Source: CAD feature listing. Evaluate the final solid. Frame: model axes, mm. A direction names the side the tool comes from. Coordinates: 2 decimals unless noted, no trailing zeros. Write each loop counter-clockwise with the first axis right and the second up, starting at its lowest first coordinate (ties: lowest second). Pieces come first, ordered by that corner, then holes. Notation, with made-up numbers: (48.25, 15.25) -> (58.25, 15.25) arc R26 cw to (58.25, 51.25) -> close; hole circle Ø2 at (-30, 77). An arc over 180 degrees is marked (long way). Write item = value, one per line.
from build123d import *

# Parameters (mm, degrees)
SKETCH1_R          = 13.5
EXTRUDE1_DEPTH     = 4
SKETCH3_R          = 10
EXTRUDE3_DEPTH     = 25
SKETCH7_R          = 8.5
CUT_EXTRUDE5_DEPTH = 16
SKETCH4_R          = 7.5
EXTRUDE4_DEPTH     = 14
CHAMFER1_SIZE      = 0.2
CHAMFER3_SIZE      = 0.3
SKETCH5_R          = 12
SKETCH5_R_2        = 10
CUT_EXTRUDE1_DEPTH = 1.5
SKETCH8_R          = 8
CUT_EXTRUDE6_DEPTH = 2
CHAMFER5_SIZE      = 1
SKETCH6_R          = 0.65
CUT_EXTRUDE2_DEPTH = 5
CHAMFER6_SIZE      = 0.2
EXTRUDE5_DEPTH     = 4


with BuildPart() as part:
    # Sketch1 → Extrude1 (new body)
    with BuildSketch(Plane.XY):
        Circle(SKETCH1_R)
    extrude(amount=EXTRUDE1_DEPTH)

    # Sketch3 → Extrude3 (add)
    with BuildSketch(Plane(origin=(0, 0, 0), x_dir=(-1, 0, 0), z_dir=(0, 0, -1))):
        Circle(SKETCH3_R)
    extrude(amount=EXTRUDE3_DEPTH)

    # Sketch7 → Cut-Extrude5 (cut)
    with BuildSketch(Plane.XY.offset(4)):
        Circle(SKETCH7_R)
    extrude(amount=-CUT_EXTRUDE5_DEPTH, mode=Mode.SUBTRACT)

    # Sketch4 → Extrude4 (add)
    with BuildSketch(Plane.XY.offset(-12)):
        Circle(SKETCH4_R)
    extrude(amount=EXTRUDE4_DEPTH)

    # Chamfer1
    chamfer1_edges = [part.edges().sort_by_distance(p)[0] for p in [
        (-7.5, 0, 2),
    ]]
    chamfer(chamfer1_edges, length=CHAMFER1_SIZE)

    # Chamfer3
    chamfer3_edges = [part.edges().sort_by_distance(p)[0] for p in [
        (-8.5, 0, 4),
        (-13.5, 0, 4),
    ]]
    chamfer(chamfer3_edges, length=CHAMFER3_SIZE)

    # Sketch5 → Cut-Extrude1 (cut)
    with BuildSketch(Plane(origin=(0, 0, 0), x_dir=(-1, 0, 0), z_dir=(0, 0, -1))):
        Circle(SKETCH5_R)
        Circle(SKETCH5_R_2, mode=Mode.SUBTRACT)
    extrude(amount=-CUT_EXTRUDE1_DEPTH, mode=Mode.SUBTRACT)

    # Sketch8 → Cut-Extrude6 (cut)
    with BuildSketch(Plane(origin=(0, 0, -25), x_dir=(-1, 0, 0), z_dir=(0, 0, -1))):
        Circle(SKETCH8_R)
    extrude(amount=-CUT_EXTRUDE6_DEPTH, mode=Mode.SUBTRACT)

    # Chamfer5
    chamfer5_edges = [part.edges().sort_by_distance(p)[0] for p in [
        (10, 0, -25),
    ]]
    chamfer(chamfer5_edges, length=CHAMFER5_SIZE)

    # Sketch6 → Cut-Extrude2 (cut)
    with BuildSketch(Plane.XY.offset(2)):
        with Locations((1.500332219, -0.655252352)):
            Circle(SKETCH6_R)
        with Locations((0, 2.126873458)):
            Circle(SKETCH6_R)
        with Locations((0, -4.848601397)):
            Circle(SKETCH6_R)
        with Locations((2.83413915, -3.376897165)):
            Circle(SKETCH6_R)
        with Locations((1.947084544, 4.606594287)):
            Circle(SKETCH6_R)
        with Locations((4.971134337, -0.373007704)):
            Circle(SKETCH6_R)
        with Locations((-4.084079731, 2.409118105)):
            Circle(SKETCH6_R)
        with Locations((-4.971134337, -0.373007704)):
            Circle(SKETCH6_R)
        with Locations((-1.947084544, 4.606594287)):
            Circle(SKETCH6_R)
        with Locations((-2.83413915, -3.376897165)):
            Circle(SKETCH6_R)
        with Locations((-1.500332219, -0.655252352)):
            Circle(SKETCH6_R)
        with Locations((4.084079731, 2.409118105)):
            Circle(SKETCH6_R)
    extrude(amount=-CUT_EXTRUDE2_DEPTH, mode=Mode.SUBTRACT)

    # Chamfer6
    chamfer6_edges = [part.edges().sort_by_distance(p)[0] for p in [
        (0.850332219, -0.655252352, 2),
        (-0.65, 2.126873458, 2),
        (-0.65, -4.848601397, 2),
        (1.297084544, 4.606594287, 2),
        (2.18413915, -3.376897165, 2),
        (4.321134337, -0.373007704, 2),
        (-4.734079731, 2.409118105, 2),
        (-5.621134337, -0.373007704, 2),
        (-2.597084544, 4.606594287, 2),
        (-3.48413915, -3.376897165, 2),
        (-2.150332219, -0.655252352, 2),
        (3.434079731, 2.409118105, 2),
    ]]
    chamfer(chamfer6_edges, length=CHAMFER6_SIZE)

    # Sketch9 → Extrude5 (add)
    with BuildSketch(Plane(origin=(0, 0, -23), x_dir=(-1, 0, 0), z_dir=(0, 0, -1))):
        Polygon((-7.216878365, 12.5), (7.216878365, 12.5), (14.43375673, 0), (7.216878365, -12.5), (-7.216878365, -12.5), (-14.43375673, 0), align=None)
    extrude(amount=-EXTRUDE5_DEPTH)


solid = part.part
1) Pull-direction query (Y, two-part tool) for faces 4 (the flat face through (7.4, -7.3, -23)), 5 (the cylindrical face through (2.17, -9.76, -23.51)), 6 (the flat face through (3, -3, -3)), 7 (the flat face through (10.775, -6.337, -21.028)); classes: +Y half, -Y half, draft (parallel to the pull), parting line (faces both ways), or undercut.
Answer block:
face_4 = draft
face_5 = parting line
face_6 = undercut
face_7 = -Y half
2) Reachability of faces 1 (the cylindrical face through (2.17, -9.76, -8.89)), 2 (the flat face through (-4, 2, -3)), 3 (the flat face through (-10.876, -6.163, -21.028)) from +Z, -Z, +X, -X, +Y, -Y: full face, straight path, thin tool, end or side. Return the list, or none.
Answer block:
face_1 = none
face_2 = +Z
face_3 = -Z, -X, -Y
3) First-contact query: pin 1 Ø12 at (y, z) = (-4.5, -10) entering from -X; pin 2 Ø2 at (x, y) = (-1.95, 4.61) entering from +Z; pin 3 Ø6 at (x, y) = (-11, 6.5) entering from -Z. Flat tips, straight axial feed; report the tip coordinate or a pass-through.
Answer block:
pin_1 = -10
pin_2 = 2
pin_3 = -24.22
4) Cut plane A-A, the plane z = -20.25. Output: boundary loops of the cut face in (x, y), and give its area (3 significant figures).
Answer block:
outline = (-14.43, 0) -> (-7.22, -12.5) -> (7.22, -12.5) -> (14.43, 0) -> (7.22, 12.5) -> (-7.22, 12.5) -> close
area = 541 mm2
5) Material intervals for probe 1 along Y at (x, z) = (-6.75, 0.25); probe 2 along Y at (x, z) = (0, -8.5); probe 3 along Z at (x, y) = (-0.5, -11.25), sorted ascending. Write a range as [from, to].
Answer block:
probe_1 = [-11.69, -9.92], [-7.38, -5.17], [-3.27, 3.27], [5.17, 7.38], [9.92, 11.69]
probe_2 = [-10, -8.5], [-7.5, 7.5], [8.5, 10]
probe_3 = [-23, -19], [1.5, 4]
